from build123d import *

# Parameters (mm, degrees)
BOSS_EXTRUDE1_DEPTH = 50.8
SKETCH2_R           = 3.175
CUT_EXTRUDE1_DEPTH  = 50.8
SKETCH6_R           = 3.175
CUT_EXTRUDE2_DEPTH  = 50.8


with BuildPart() as part:
    # Sketch1 → Boss-Extrude1 (new body)
    with BuildSketch(Plane(origin=(0, 0, 0), x_dir=(0, 0, -1), z_dir=(1, 0, 0))):
        Polygon((-29.265887299, 19.069791765), (-29.265887299, -31.730208235), (21.534112701, -31.730208235), (21.534112701, 19.069791765), (18.359112701, 19.069791765), (18.359112701, -28.555208235), (-26.090887299, -28.555208235), (-26.090887299, 19.069791765), align=None)
    extrude(amount=BOSS_EXTRUDE1_DEPTH)

    # Sketch2 → Cut-Extrude1 (cut)
    with BuildSketch(Plane(origin=(0, 0, -21.534112701), x_dir=(-1, 0, 0), z_dir=(0, 0, -1))):
        with Locations((-38.1, 12.680491765)):
            Circle(SKETCH2_R)
        with Locations((-7.8232, 12.680491765)):
            Circle(SKETCH2_R)
    extrude(amount=-CUT_EXTRUDE1_DEPTH, mode=Mode.SUBTRACT)

    # Sketch6 → Cut-Extrude2 (cut)
    with BuildSketch(Plane.XZ.offset(31.730208235)):
        with Locations(Location((41.275, 3.865887299, 0), (0, 0, 270))):
            Circle(SKETCH6_R)
        with Locations(Location((25.4, 3.865887299, 0), (0, 0, 270))):
            Circle(SKETCH6_R)
        with Locations(Location((9.525, 3.865887299, 0), (0, 0, 270))):
            Circle(SKETCH6_R)
    extrude(amount=-CUT_EXTRUDE2_DEPTH, mode=Mode.SUBTRACT)


solid = part.part
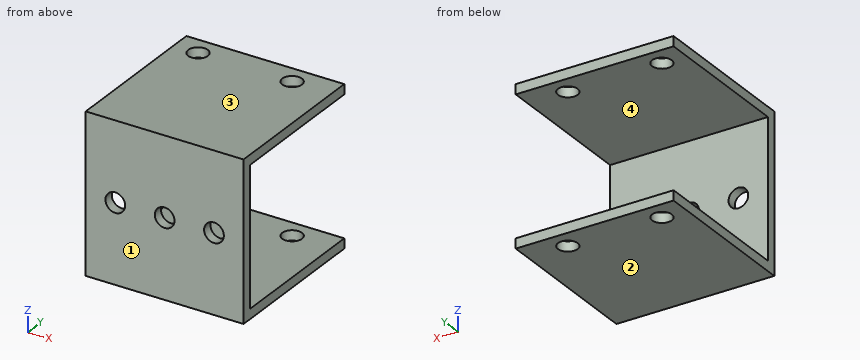
Could you check a few things on this model? Use its own coordinates, in mm. Face numbers are marked on the shaded views. Round coordinates to 2 decimals unless told otherwise and drop trailing zeros. Order: outer loops, then holes, each group sorted by start corner. A loop starts at its lowest first (then second) coordinate and runs counter-clockwise, first axis right, second up.
(1) Imagine slicing it at B-B (y = -2). Write out the boundary of the cut face in (x, z), plus the area to 3 significant figures.
Response values:
outline: (0, -21.53) - (50.8, -21.53) - (50.8, -18.36) - (0, -18.36) - close; (0, 26.09) - (50.8, 26.09) - (50.8, 29.27) - (0, 29.27) - close
area: 323 mm2
(2) If we mould it in two halves opening along Z, with no side actions, what happens to the marked faces 1, 2, 3 and 4? For each: released by +Z, released by -Z, zero draft, split by the parting line, or undercut.
Response values:
face 1: zero draft
face 2: released by -Z
face 3: released by +Z
face 4: undercut
(3) I'm going to push flat-ended pins straight in: pin 1 (10 mm diameter, centred on x = 38.1, y = 12.68, fed in from +Z); pin 2 (4 mm diameter, centred on x = 41.28, z = 3.87, fed in from -Y); pin 3 (13.5 mm diameter, centred on x = 26.5, z = 5.5, fed in from +Y). Where does each tip first touch, or does it pass through?
Response values:
pin 1: stops at z = 29.27
pin 2: passes through
pin 3: stops at y = -28.56
(4) Imagine slicing it at A-A (x = 25.4). Write out the boundary of the cut face in (y, z).
Response values:
outline: (-31.73, -21.53) - (19.07, -21.53) - (19.07, -18.36) - (-28.56, -18.36) - (-28.56, 0.69) - (-31.73, 0.69) - close; (-31.73, 7.04) - (-28.56, 7.04) - (-28.56, 26.09) - (19.07, 26.09) - (19.07, 29.27) - (-31.73, 29.27) - close
(5) Imagine slicing it at C-C (z = 2.5). Write out the boundary of the cut face in (x, y), plus the area to 3 significant figures.
Response values:
outline: (0, -31.73) - (6.66, -31.73) - (6.66, -28.56) - (0, -28.56) - close; (12.39, -31.73) - (22.53, -31.73) - (22.53, -28.56) - (12.39, -28.56) - close; (28.27, -31.73) - (38.41, -31.73) - (38.41, -28.56) - (28.27, -28.56) - close; (44.14, -31.73) - (50.8, -31.73) - (50.8, -28.56) - (44.14, -28.56) - close
area: 107 mm2
(6) Imagine slicing it at D-D (z = -7). Write out the boundary of the cut face in (x, y).
Response values:
outline: (0, -31.73) - (50.8, -31.73) - (50.8, -28.56) - (0, -28.56) - close
(7) Please list where these lines run through material, in increasing order: line 1 along Z through (x, y) = (13.5, 15); line 2 along Y through (x, z) = (38, 27); line 3 along Y through (x, z) = (21.5, -14).
Response values:
line 1: z = -21.53 to -18.36, 26.09 to 29.27
line 2: y = -31.73 to 9.51, 15.85 to 19.07
line 3: y = -31.73 to -28.56
